Geometry check sheet. Reference: the model listing, model coordinates, mm. A direction names the side the tool comes from. Give positions to 0.01 mm unless a question says otherwise; leave off trailing zeros. Write each loop counter-clockwise with the first axis right and the second up, starting at its lowest first coordinate (ties: lowest second). Pieces come first, ordered by that corner, then holes. Notation, with made-up numbers: (-1.5, -26.75) - (47.5, -26.75) arc R24 cw to (47.5, 7.25) - close; hole circle Ø2 at (77, 52.5). An arc over 180 degrees is marked (long way). One line per question, with ' | ' between items. Start each with the question number.
Q1. Section check C-C on z = 2.25. Record the boundary of the cut face in (x, y).
Q2. Gauge pin test, flat ends, axial feed: P1, Ø25, axis at x = 0, y = 0, coming from the +Z side; P2, Ø1, axis at y = -20.5, z = 6.5, coming from the +X side; P3, Ø3, axis at x = -35, y = 0, coming from the +Z side; P4, Ø2, axis at y = -5.5, z = 3, coming from the -X side. Record the tip position at first contact, or that the pin passes through.
Q3. Thickness scan on L1, parallel to Y at x = 0, z = 4.5; L2, parallel to Y at x = 0, z = 1.35; L3, parallel to Y at x = 7, z = 5.75. Record the ranges inside material, lowest first. Write a range as [from, to].
Q4. Section check D-D on x = -13. Record the boundary of the cut face in (y, z), and give its area (3 significant figures).
Q5. Release check for a two-part mould opening along Y. For faces 4 (the face through (35.102, -14.554, 3.944)), 5 (the face through (16, 1, 0)), 6 (the face through (-3.01, -13.57, 5.97)) record: +Y half, -Y half, draft (parallel to the pull), parting line (faces both ways), or undercut.
Q6. Section check A-A on x = 0. Record the boundary of the cut face in (y, z), and give its area (3 significant figures).
Q7. Set-up check for faces 1 (the face through (-0.74, -36.92, 2.27)), 2 (the face through (6.691, -12.864, 1.972)), 3 (the face through (32.5, 0.1, 6.3)): record each of +Z, -Z, +X, -X, +Y, -Y from which the full face is reachable in a straight line by a thin tool's end or side.
Q8. Section check B-B on y = -35.5. Record the boundary of the cut face in (x, z), and give its area (3 significant figures).
```python
from build123d import *

# Parameters (mm, degrees)
SKETCH_1_R                = 38
SKETCH_1_R_2              = 13.9
EXTRUDE_1_DEPTH           = 8
HOLE_WIZARD_1_D           = 3.2
HOLE_WIZARD_1_CBORE_D     = 6
HOLE_WIZARD_1_CBORE_DEPTH = 3.4
HOLE_WIZARD_4_0_4_1_D     = 4
CHAMFER_1_SIZE            = 1
SKETCH_9_R                = 14.5
CUT_EXTRUDE_1_DEPTH       = 4


with BuildPart() as part:
    # 草图1 → 凸台-拉伸1 (new body)
    with BuildSketch(Plane.XY):
        Circle(SKETCH_1_R)
        Circle(SKETCH_1_R_2, mode=Mode.SUBTRACT)
    extrude(amount=EXTRUDE_1_DEPTH)

    # 打孔尺寸(%根据)内六角圆柱头螺钉的类型1 (through all)
    with Locations(Plane.XY.offset(8)):
        with Locations((0, 35.5), (35.5, 0), (0, -35.5), (-35.5, 0)):
            CounterBoreHole(HOLE_WIZARD_1_D / 2, HOLE_WIZARD_1_CBORE_D / 2, HOLE_WIZARD_1_CBORE_DEPTH)

    # Ø4.0 (4) 直径孔1 (through all)
    with Locations(Plane(origin=(0, 0, 0), x_dir=(-1, 0, 0), z_dir=(0, 0, -1))):
        with Locations((27.9, 0)):
            Hole(HOLE_WIZARD_4_0_4_1_D / 2)

    # 倒角1
    chamfer_1_edges = [part.edges().sort_by_distance(p)[0] for p in [
        (-29.9, 0, 0),
        (-29.9, 0, 8),
    ]]
    chamfer(chamfer_1_edges, length=CHAMFER_1_SIZE)

    # 草图9 → 切除-拉伸1 (cut)
    with BuildSketch(Plane.XY):
        Circle(SKETCH_9_R)
    extrude(amount=CUT_EXTRUDE_1_DEPTH, mode=Mode.SUBTRACT)


solid = part.part
```
Working result:
1) outline: circle Ø76 at (0, 0); hole circle Ø3.2 at (-35.5, 0); hole circle Ø4 at (-27.9, 0); hole circle Ø29 at (0, 0); hole circle Ø3.2 at (0, -35.5); hole circle Ø3.2 at (0, 35.5); hole circle Ø3.2 at (35.5, 0)
2) P1: passes through | P2: stops at x = 32.31 | P3: stops at z = 4.6 | P4: stops at x = -37.73
3) L1: y = [-38, -37.1], [-33.9, -13.9], [13.9, 33.9], [37.1, 38] | L2: y = [-38, -37.1], [-33.9, -14.5], [14.5, 33.9], [37.1, 38] | L3: y = [-37.35, -12.01], [12.01, 37.35]
4) outline: (-35.71, 0) - (-6.42, 0) - (-6.42, 4) - (-4.92, 4) - (-4.92, 8) - (-35.71, 8) - close; (4.92, 4) - (6.42, 4) - (6.42, 0) - (35.71, 0) - (35.71, 8) - (4.92, 8) - close | area: 481 mm2
5) face 4: parting line | face 5: draft | face 6: undercut
6) outline: (-38, 0) - (-37.1, 0) - (-37.1, 4.6) - (-38, 4.6) - close; (-33.9, 0) - (-14.5, 0) - (-14.5, 4) - (-13.9, 4) - (-13.9, 8) - (-32.5, 8) - (-32.5, 4.6) - (-33.9, 4.6) - close; (13.9, 4) - (14.5, 4) - (14.5, 0) - (33.9, 0) - (33.9, 4.6) - (32.5, 4.6) - (32.5, 8) - (13.9, 8) - close; (37.1, 0) - (38, 0) - (38, 4.6) - (37.1, 4.6) - close | area: 314 mm2
7) face 1: +Z, -Z | face 2: -Z | face 3: +Z
8) outline: (-13.56, 0) - (-1.6, 0) - (-1.6, 4.6) - (-3, 4.6) - (-3, 8) - (-13.56, 8) - close; (1.6, 0) - (13.56, 0) - (13.56, 8) - (3, 8) - (3, 4.6) - (1.6, 4.6) - close | area: 182 mm2
